Verification items for this drawing (mm, ordinates from the low corner). A direction names the side the tool comes from. Round coordinates to 2 decimals unless told otherwise and drop trailing zeros. Write each loop counter-clockwise with the first axis right and the second up, starting at its lowest first coordinate (ties: lowest second). Pieces come first, ordered by that corner, then holes.
Item 1: Depth check by flat-ended pin: P1, Ø12, axis at x = 34.5, z = 28.5, coming from the -Y side; P2, Ø5, axis at x = 33.5, z = 25.5, coming from the +Y side; P3, Ø2.5, axis at x = 29.5, y = 2, coming from the +Z side. Enter the tip coordinate at first touch or a pass-through.
Item 2: Draft check along Z on the marked faces 1, 2, 3 and 4. Enter one of: pulls with the +Z half, pulls with the -Z half, needs draft (parallel to the pull), parting line crosses it, or undercut.
Item 3: Cross-section at A-A (y = 12.7). State how many separate pieces and enclosed holes the cut face has, then the cut area to 3 significant figures.
Item 4: Scan lines: probe 1 along Y at (x, z) = (44.45, 8); probe 2 along Y at (x, z) = (51.5, 3.5) (1 decimal); probe 3 along X at (y, z) = (12.25, 32). Record each from-to range of solid material in increasing order.
Item 5: Cross-section at C-C (x = 18.5). Enter the section's corners in (y, z) (1 decimal), then the cut area to 3 significant figures.
Item 6: Access from +Z, -Z, +X, -X, +Y, -Y to the whole of each face (thin tool, end or side, straight path). Record for the marked faces 5, 6 and 7.
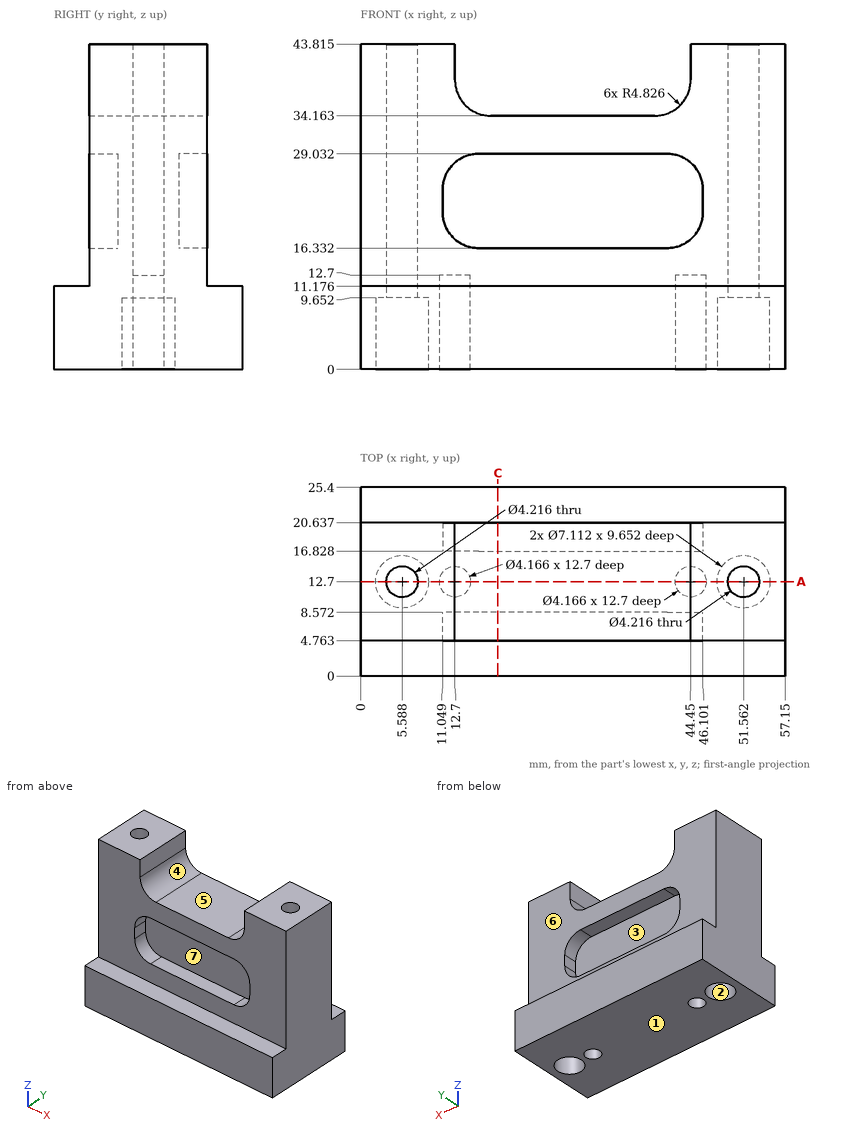
Resolved:
1. P1: stops at y = 4.76
1. P2: stops at y = 16.83
1. P3: stops at z = 11.18
2. face 1: pulls with the -Z half
2. face 2: needs draft
2. face 3: undercut
2. face 4: pulls with the +Z half
3. separate pieces: 3
3. enclosed holes: 0
3. area: 1,680 mm2
4. probe 1: y = 0 to 10.62, 14.78 to 25.4
4. probe 2: y = 0 to 9.1, 16.3 to 25.4
4. probe 3: x = 0 to 3.53, 7.65 to 49.5, 53.62 to 57.15
5. outline: (0, 0) - (25.4, 0) - (25.4, 11.2) - (20.6, 11.2) - (20.6, 16.3) - (16.8, 16.3) - (16.8, 29) - (20.6, 29) - (20.6, 34.2) - (4.8, 34.2) - (4.8, 29) - (8.6, 29) - (8.6, 16.3) - (4.8, 16.3) - (4.8, 11.2) - (0, 11.2) - close
5. area: 552 mm2
6. face 5: +Z, +Y, -Y
6. face 6: +Z, +X, -X, +Y
6. face 7: -Y
